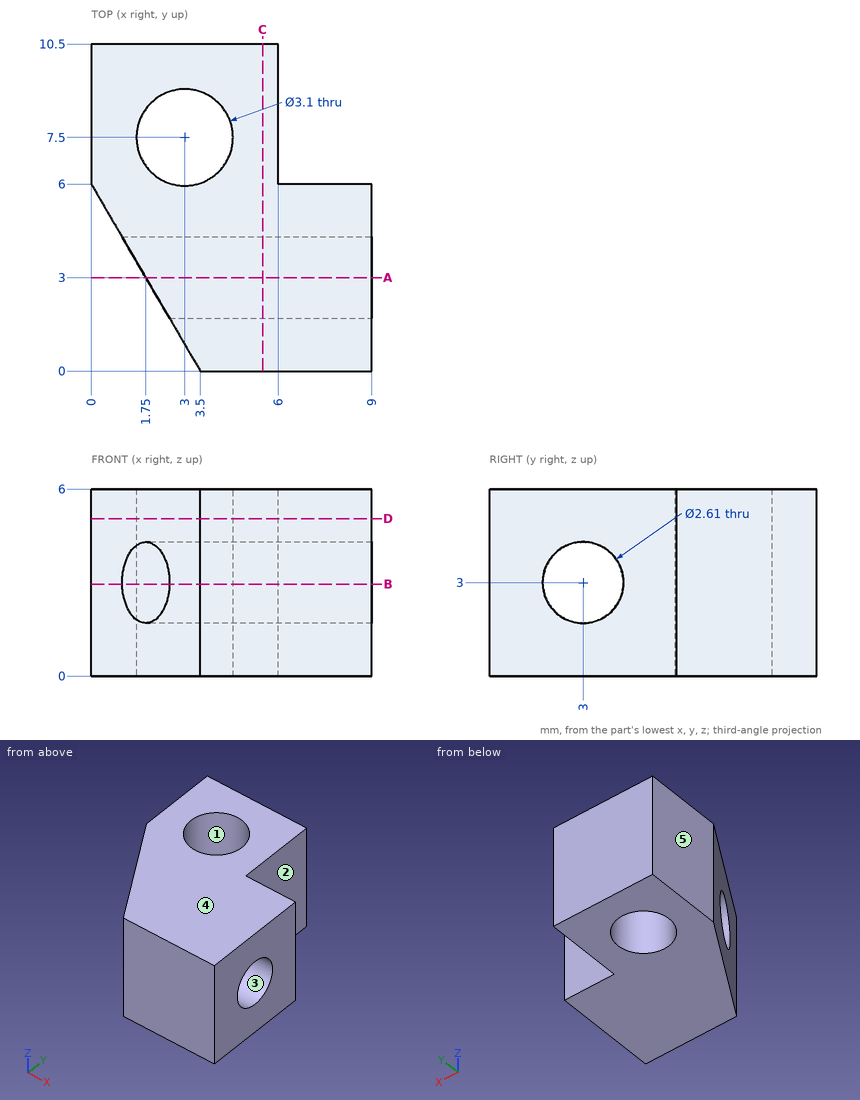
Drawing for the job (mm, zero at the part's lowest x, y, z). A direction names the side the tool comes from. Coordinates: 2 decimals unless noted, no trailing zeros. Order: outer loops, then holes, each group sorted by start corner. A loop starts at its lowest first (then second) coordinate and runs counter-clockwise, first axis right, second up.
Item 1: Pin check, flat tips, straight feed: pin 1 Ø0.9 at (x, z) = (7, 2.5) entering from +Y; pin 2 Ø1.3 at (y, z) = (8.5, 1.5) entering from +X. Stop position of each tip, or through.
Check sheet entries:
pin 1: stops at y = 6
pin 2: stops at x = 6
Item 2: Band-saw the part on C-C on x = 5.5. List the corners of the cut face in (y, z) (3 decimals), plus the area to 3 significant figures.
Check sheet entries:
outline: (0, 0) - (10.5, 0) - (10.5, 6) - (0, 6) - close; hole circle Ø2.61 at (3, 3)
area: 57.6 mm2
Item 3: 3-axis set-ups, long thin cutter, end or side, ignore diameter. For the marked faces 1 and 2: which of +Z, -Z, +X, -X, +Y, -Y reach the whole face in a straight line?
Check sheet entries:
face 1: +Z, -Z
face 2: +Z, -Z, +X, +Y
Item 4: Band-saw the part on D-D on z = 5.05. List the corners of the cut face in (x, y).
Check sheet entries:
outline: (0, 6) - (3.5, 0) - (9, 0) - (9, 6) - (6, 6) - (6, 10.5) - (0, 10.5) - close; hole circle Ø3.1 at (3, 7.5)
Item 5: Band-saw the part on B-B on z = 2.95. List the corners of the cut face in (x, y), plus the area to 3 significant figures.
Check sheet entries:
outline: (0, 6) - (0.99, 4.3) - (9, 4.3) - (9, 6) - (6, 6) - (6, 10.5) - (0, 10.5) - close; (2.51, 1.7) - (3.5, 0) - (9, 0) - (9, 1.7) - close; hole circle Ø3.1 at (3, 7.5)
area: 44.0 mm2
Item 6: Drill centre lines: L1, parallel to Y at x = 4, z = 2.2; L2, parallel to Z at x = 6.5, y = 3 (3 decimals); L3, parallel to Y at x = 3, z = 3 (3 decimals). Where is each one in solid material? Low to high.
Check sheet entries:
L1: y = 0 to 1.97, 4.03 to 6.32, 8.68 to 10.5
L2: z = 0 to 1.695, 4.305 to 6
L3: y = 0.857 to 1.695, 4.305 to 5.95, 9.05 to 10.5
Item 7: Two-plate mould, pull along Z, no slides. Class the marked faces 3, 4 and 5: +Z half, -Z half, draft (parallel to the pull), parting line (faces both ways), or undercut.
Check sheet entries:
face 3: undercut
face 4: +Z half
face 5: draft
Item 8: Band-saw the part on A-A on y = 3. List the corners of the cut face in (x, z) (3 decimals), plus the area to 3 significant figures.
Check sheet entries:
outline: (1.75, 0) - (9, 0) - (9, 1.695) - (1.75, 1.695) - close; (1.75, 4.305) - (9, 4.305) - (9, 6) - (1.75, 6) - close
area: 24.6 mm2
